Input: part model. Units: mm. Frame: model coordinates. Coordinates: 2 decimals unless noted, no trailing zeros. Write each loop counter-clockwise with the first axis right and the second up, starting at its lowest first coordinate (ties: lowest second). Pieces come first, ordered by that corner, then holes. Notation, with made-up numbers: (50, 26.5) - (83, 26.5) arc R29 ccw to (83, 53.5) - close; hole circle Ø11 at (-15, 41). An arc over 180 degrees is marked (long way). Put each result on its own line as item: value. Start each with the question number.
1. Cut plane C-C, the plane z = 7. Return loops of the section in (x, y).
2. Cut plane D-D, the plane z = 27.5. Return loops of the section in (x, y).
3. Pin query (flat end, axial travel): pin 1 (1 mm diameter, centred on x = 6.5, z = 13, fed in from -Y); pin 2 (3 mm diameter, centred on y = 6.5, z = 13, fed in from +X); pin 3 (5 mm diameter, centred on x = -1.5, z = 26, fed in from -Y). Return the tip coordinate at first contact, or that it passes through.
4. Line query: line 1 (X direction, y = 0.5, z = 12.5); line 2 (Z direction, x = 6.5, y = 5.75); line 3 (X direction, y = -7.5, z = -13.5). Output: solid intervals per line, ascending.
5. Cut plane A-A, the plane x = 0. Return loops of the section in (y, z), and give its area (3 significant figures).
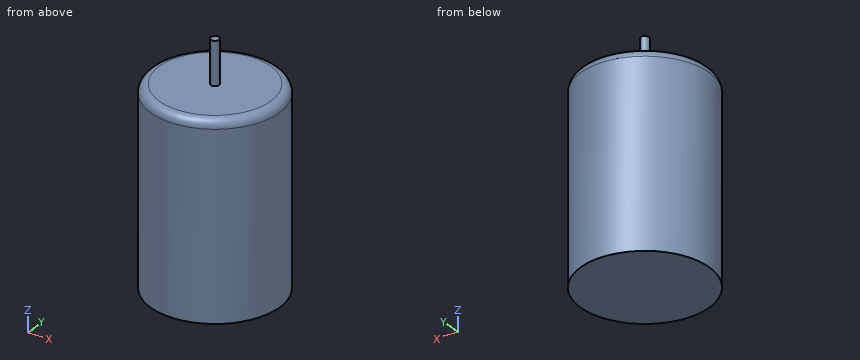
Solid Edge part; units mm, degrees
sketch "Sketch1" plane through (0, 0, 0) normal (0, 0, 1) x (1, 0, 0)
  circle A0 centre (0, 0) radius 15
extrude "Ajout_matière_1" add sketch "Sketch1" along normal mid plane 45
sketch "Sketch2" plane through (0, 0, 22.5) normal (0, 0, 1) x (1, 0, 0)
  circle A0 centre (0, 0) radius 1
extrude "Ajout_matière_2" add sketch "Sketch2" along normal blind 10
fillet "Congé_1" radius 2 1 edges at (-15, 0, 22.5)
properties material "Acier S235"
Report:
1. outline: circle Ø30 at (0, 0)
2. outline: circle Ø2 at (0, 0)
3. pin 1: stops at y = -13.75
3. pin 2: stops at x = 14.14
3. pin 3: stops at y = -1
4. line 1: x = -14.99 to 14.99
4. line 2: z = -22.5 to 22.5
4. line 3: x = -12.99 to 12.99
5. outline: (-15, -22.5) - (15, -22.5) - (15, 20.5) arc R2 ccw to (13, 22.5) - (1, 22.5) - (1, 32.5) - (-1, 32.5) - (-1, 22.5) - (-13, 22.5) arc R2 ccw to (-15, 20.5) - close
5. area: 1,370 mm^2
